Build history of the part. All positions in model axes, mm. A direction names the side the tool comes from. Round coordinates to 2 decimals unless told otherwise and drop trailing zeros. Order: outer loops, then holes, each group sorted by start corner. A loop starts at its lowest first (then second) coordinate and runs counter-clockwise, first axis right, second up. Notation, with made-up numbers: (-8.75, 12.25) -> (45.25, 12.25) arc R20 ccw to (45.25, 38.25) -> close; hole circle Ø9 at (35.5, -40). An arc over 180 degrees is marked (long way). Answer as CSV lines item,"result". Start each with the question number.
```python
from build123d import *

# Parameters (mm, degrees)
SKETCH2_R           = 2.5
BOSS_EXTRUDE1_DEPTH = 6.35


with BuildPart() as part:
    # Sketch2 → Boss-Extrude1 (new, symmetric)
    with BuildSketch(Plane(origin=(0, 0, 0), x_dir=(1, 0, 0), z_dir=(0, 1, 0))):
        with BuildLine():
            Line((-34.883854573, -4.808079014), (-14.712038095, 12.5))
            Line((-14.712038095, 12.5), (20, 12.5))
            Line((20, 12.5), (20, -12.5))
            Line((20, -12.5), (0, -12.5))
            Line((0, -12.5), (-28.616418364, -17.871275457))
            ThreePointArc((-28.616418364, -17.871275457), (-36.762008058, -13.74426371), (-34.883854573, -4.808079014))
        make_face()
        with Locations(Location((-30, -10.5, 0), (0, 0, 270))):
            Circle(SKETCH2_R, mode=Mode.SUBTRACT)
        Polygon((-21.542043285, 0.051346502), (-21.542043285, -0.051346502), (10, -5.61305976), (10, 5.61305976), align=None, mode=Mode.SUBTRACT)
    extrude(amount=BOSS_EXTRUDE1_DEPTH, both=True)


solid = part.part
```
Q1. Flat gauge pins, fed straight in: pin 1 Ø1.5 at (y, z) = (-1.5, 4.5) entering from -X; pin 2 Ø4 at (x, y) = (8, 1) entering from +Z; pin 3 Ø6 at (x, y) = (-23, 1) entering from +Z. Where does each tip first touch, or does it go through?
Q2. Two-plate mould, pull along Z, no slides. Class faces 3 (the face through (10, 0, 12.5)), 4 (the face through (-27.52, -0.09, 10.17)), 5 (the face through (-24.939, 0.089, -3.725)): +Z half, -Z half, draft (parallel to the pull), parting line (faces both ways), or undercut.
Q3. Slice it at D-D, the plane x = 12. Write the cut outline in (y, z).
Q4. Probe L1, parallel to X at y = -1, z = 10.5; L2, parallel to Z at x = 5, y = -1.5; L3, parallel to X at y = -2, z = 10. List the from-to ranges inside material, lowest first.
Q5. Slice it at A-A, the plane z = 10.5. Write the cut outline in (x, y), plus the area to 3 significant figures.
Q6. Which spindle directions (+Z, -Z, +X, -X, +Y, -Y) get a long thin tool onto all of the face, cutting with end or side? Do faces 1 (the face through (-8, -6.35, 3)), 2 (the face through (-5.992, 0.089, 2.793)). Say none if no direction does.
Q7. Slice it at C-C, the plane y = -5.5. Write the cut outline in (x, z), plus the area to 3 significant figures.
Q8. Slice it at B-B, the plane x = 6. Write the cut outline in (y, z).
Solutions:
1,pin 1,"stops at x = -35.36"
1,pin 2,"stops at z = 12.5"
1,pin 3,"stops at z = 17.38"
2,face 3,"+Z half"
2,face 4,"undercut"
2,face 5,"-Z half"
3,outline,"(-6.35, -12.5) -> (6.35, -12.5) -> (6.35, 12.5) -> (-6.35, 12.5) -> close"
4,L1,"x = -37.5 to -32.5, -27.5 to 20"
4,L2,"z = -12.5 to -4.73, 4.73 to 12.5"
4,L3,"x = -37.48 to -32.45, -27.55 to 20"
5,outline,"(-37.5, -6.35) -> (-32.5, -6.35) -> (-32.5, 6.35) -> (-37.5, 6.35) -> close; (-27.5, -6.35) -> (20, -6.35) -> (20, 6.35) -> (-27.5, 6.35) -> close"
5,area,"667 mm2"
6,face 1,"+Z, -Z, +X, -X, -Y"
6,face 2,"+Y, -Y"
7,outline,"(-34.88, 4.81) -> (-14.71, -12.5) -> (20, -12.5) -> (20, 12.5) -> (0, 12.5) -> (-28.62, 17.87) arc R7.5 ccw to start; hole circle Ø5 at (-30, 10.5); hole (-21.54, -0.05) -> (10, -5.61) -> (10, 5.61) -> (-21.54, 0.05) -> close"
7,area,"1,130 mm2"
8,outline,"(-6.35, -12.5) -> (6.35, -12.5) -> (6.35, -4.91) -> (-6.35, -4.91) -> close; (-6.35, 4.91) -> (6.35, 4.91) -> (6.35, 12.5) -> (-6.35, 12.5) -> close"
